Can you work these out from the model? Positions are in its coordinate system, mm. A direction names the side the tool comes from. Coordinates: 2 decimals unless noted, no trailing zeros. Write each loop counter-clockwise with the first axis right and the second up, starting at its lowest first coordinate (ties: lowest second). Pieces come first, ordered by that corner, then holes. Notation, with made-up numbers: (22, -34.5) -> (71, -34.5) arc R14 ccw to (71, -7.5) -> close; hole circle Ø4 at (72.25, 42). An arc over 180 degrees is marked (long way). Use one line per item in the form item = value.
```python
from build123d import *

# Parameters (mm, degrees)
SKETCH1_W           = 8
SKETCH1_H           = 2.5
BOSS_EXTRUDE1_DEPTH = 9
SKETCH2_R           = 1.55
CUT_EXTRUDE1_DEPTH  = 3.5


with BuildPart() as part:
    # Sketch1 → Boss-Extrude1 (new body)
    with BuildSketch(Plane.XY):
        with Locations((4, -1.25)):
            Rectangle(SKETCH1_W, SKETCH1_H)
        Polygon((0, -7.7), (0, 0), (-2.5, 0), (-2.5, -5.3), (-3.3, -6.1), (-3.3, -7.7), align=None)
    extrude(amount=BOSS_EXTRUDE1_DEPTH)

    # Sketch2 → Cut-Extrude1 (cut, through all)
    with BuildSketch(Plane.XZ.offset(2.5)):
        with Locations((4, 4.5)):
            Circle(SKETCH2_R)
    extrude(amount=-CUT_EXTRUDE1_DEPTH, mode=Mode.SUBTRACT)


solid = part.part
```
Q1. Suppose I cut it at B-B (z = 4.5). Write out the boundary of the cut face in (x, y), then the cut area to 3 significant figures.
Return value:
outline = (-3.3, -7.7) -> (0, -7.7) -> (0, -2.5) -> (2.45, -2.5) -> (2.45, 0) -> (-2.5, 0) -> (-2.5, -5.3) -> (-3.3, -6.1) -> close; (5.55, -2.5) -> (8, -2.5) -> (8, 0) -> (5.55, 0) -> close
area = 33.1 mm2
Q2. Suppose I cut it at A-A (x = 4). Write out the boundary of the cut face in (y, z), then the cut area to 4 significant figures.
Return value:
outline = (-2.5, 0) -> (0, 0) -> (0, 2.95) -> (-2.5, 2.95) -> close; (-2.5, 6.05) -> (0, 6.05) -> (0, 9) -> (-2.5, 9) -> close
area = 14.75 mm2
Q3. If I drill on line 1 (Y direction, x = 7.25, z = 4); line 2 (Z direction, x = 4, y = -1.6), over which ranges is the centre line in solid material (lowest first)? Write a range as from..to.
Return value:
line_1 = -2.5..0
line_2 = 0..2.95, 6.05..9
Q4. For faces 5 (the flat face through (-2.5, -3, 4)), 6 (the flat face through (-3.3, -7, 4)), 7 (the flat face through (0, -5, 4)), which set-ups out of +Z, -Z, +X, -X, +Y, -Y let a thin tool reach every point of the face, with its end or its side?
Return value:
face_5 = +Z, -Z, -X, +Y
face_6 = +Z, -Z, -X, +Y, -Y
face_7 = +Z, -Z, +X, -Y
Q5. Will these pins go through, and if not, where does the flat tip stop? pin 1 (1.9 mm diameter, centred on x = 4, z = 4.5, fed in from +Y) (3 decimals); pin 2 (5 mm diameter, centred on x = 6.5, z = 3.5, fed in from -Y); pin 3 (2.5 mm diameter, centred on y = -5.5, z = 5.5, fed in from +X).
Return value:
pin_1 = through
pin_2 = -2.5
pin_3 = 0
Q6. Suppose I cut it at D-D (x = 6.5). Write out the boundary of the cut face in (y, z), then the cut area to 3 significant figures.
Return value:
outline = (-2.5, 0) -> (0, 0) -> (0, 9) -> (-2.5, 9) -> close
area = 22.5 mm2
Q7. Suppose I cut it at C-C (z = 7.25). Write out the boundary of the cut face in (x, y).
Return value:
outline = (-3.3, -7.7) -> (0, -7.7) -> (0, -2.5) -> (8, -2.5) -> (8, 0) -> (-2.5, 0) -> (-2.5, -5.3) -> (-3.3, -6.1) -> close
Q8. Thinking about a two-plate mould opening in Z: for faces 1 (the cylindrical face through (2.45, -1.27, 4.57)), 2 (the flat face through (1, -2, 9)), 3 (the flat face through (1, -2, 0)), 4 (the flat face through (3, 0, 3)), which applies, released by +Z, released by -Z, zero draft, split by the parting line, or undercut?
Return value:
face_1 = undercut
face_2 = released by +Z
face_3 = released by -Z
face_4 = zero draft
